from build123d import *

# Parameters (mm, degrees)
F0_W     = 22
F0_H     = 22
F1_DEPTH = 4
F3_R     = 1.35
F4_DEPTH = 4.001
F5_W     = 6
F5_H     = 12
F6_DEPTH = 4.001
F5_R     = 8
F7_DEPTH = 3


with BuildPart() as f1:
    # F0 (on Top) → F1 (new body)
    with BuildSketch(Plane.XY):
        with Locations((11, 11)):
            Rectangle(F0_W, F0_H)
    extrude(amount=F1_DEPTH)

    # F3 (on face) → F4 (cut, through all)
    with BuildSketch(Plane.XY.offset(4)):
        with Locations((3, 3)):
            Circle(F3_R)
        with Locations((3, 19)):
            Circle(F3_R)
        with Locations((19, 3)):
            Circle(F3_R)
        with Locations((19, 19)):
            Circle(F3_R)
    extrude(amount=-F4_DEPTH, mode=Mode.SUBTRACT)

    # F5 (on face) → F6 (cut, through all)
    with BuildSketch(Plane.XY.offset(4)):
        with Locations((11, 11)):
            Rectangle(F5_W, F5_H)
    extrude(amount=-F6_DEPTH, mode=Mode.SUBTRACT)

    # F5 (on face) → F7 (cut, through all)
    with BuildSketch(Plane.XY.offset(4)):
        with Locations((11, 11)):
            Circle(F5_R)
        with Locations((11, 11)):
            Rectangle(F5_W, F5_H, mode=Mode.SUBTRACT)
    extrude(amount=-F7_DEPTH, mode=Mode.SUBTRACT)


solid = f1.part
Here's how the part is built. I have some questions about the finished solid (model axes, mm). A direction names the side the tool comes from. Give positions to 0.01 mm unless a question says otherwise; leave off trailing zeros. Order: outer loops, then holes, each group sorted by start corner. A loop starts at its lowest first (then second) coordinate and runs counter-clockwise, first axis right, second up. Notation, with made-up numbers: (28, 9) -> (86, 9) arc R17 cw to (86, 35) -> close; hole circle Ø1 at (36.25, 73). An arc over 180 degrees is marked (long way). One line per item, written item: value. Start each with the question number.
1. Imagine slicing it at C-C, the plane y = 11. List the corners of the cut face in (x, z) for me.
2. I need wall thicknesses on probe 1 along X at (y, z) = (9.5, 0.7); probe 2 along Y at (x, z) = (11, 1.75); probe 3 along X at (y, z) = (2, 0.4). Which ranges of each line are inside material? Lowest first, please. Write a range as from..to.
3. We'd pull the mould along Y, two halves only. Please class faces 4 (the face through (0, 11, 2)), 5 (the face through (11, 0, 2)), 6 (the face through (11, 5, 0.5)): released by +Y, released by -Y, zero draft, split by the parting line, or undercut.
4. Imagine slicing it at A-A, the plane x = 11. List the corners of the cut face in (y, z) for me.
5. Imagine slicing it at D-D, the plane z = 0.45. List the corners of the cut face in (x, y) for me.
6. Imagine slicing it at B-B, the plane z = 2.2. List the corners of the cut face in (x, y) for me.
7. For faces 1 (the face through (9.27, 3.19, 2.52)), 2 (the face through (11, 22, 2)), 3 (the face through (8, 10.9, 0.5)), which set-ups out of +Z, -Z, +X, -X, +Y, -Y let a thin tool reach every point of the face, with its end or its side?
8. Will these pins go through, and if not, where does the flat tip stop? pin 1 Ø2 at (x, y) = (19, 19) entering from +Z; pin 2 Ø8 at (x, y) = (12.5, 14.5) entering from +Z.
Values follow:
1. outline: (0, 0) -> (8, 0) -> (8, 1) -> (3, 1) -> (3, 4) -> (0, 4) -> close; (14, 0) -> (22, 0) -> (22, 4) -> (19, 4) -> (19, 1) -> (14, 1) -> close
2. probe 1: x = 0..8, 14..22
2. probe 2: y = 0..3, 19..22
2. probe 3: x = 0..2.09, 3.91..18.09, 19.91..22
3. face 4: zero draft
3. face 5: released by -Y
3. face 6: undercut
4. outline: (0, 0) -> (5, 0) -> (5, 1) -> (3, 1) -> (3, 4) -> (0, 4) -> close; (17, 0) -> (22, 0) -> (22, 4) -> (19, 4) -> (19, 1) -> (17, 1) -> close
5. outline: (0, 0) -> (22, 0) -> (22, 22) -> (0, 22) -> close; hole circle Ø2.7 at (3, 3); hole circle Ø2.7 at (3, 19); hole (8, 5) -> (14, 5) -> (14, 17) -> (8, 17) -> close; hole circle Ø2.7 at (19, 3); hole circle Ø2.7 at (19, 19)
6. outline: (0, 0) -> (22, 0) -> (22, 22) -> (0, 22) -> close; hole circle Ø2.7 at (3, 3); hole circle Ø2.7 at (3, 19); hole circle Ø16 at (11, 11); hole circle Ø2.7 at (19, 3); hole circle Ø2.7 at (19, 19)
7. face 1: +Z
7. face 2: +Z, -Z, +X, -X, +Y
7. face 3: +Z, -Z
8. pin 1: passes through
8. pin 2: stops at z = 1
